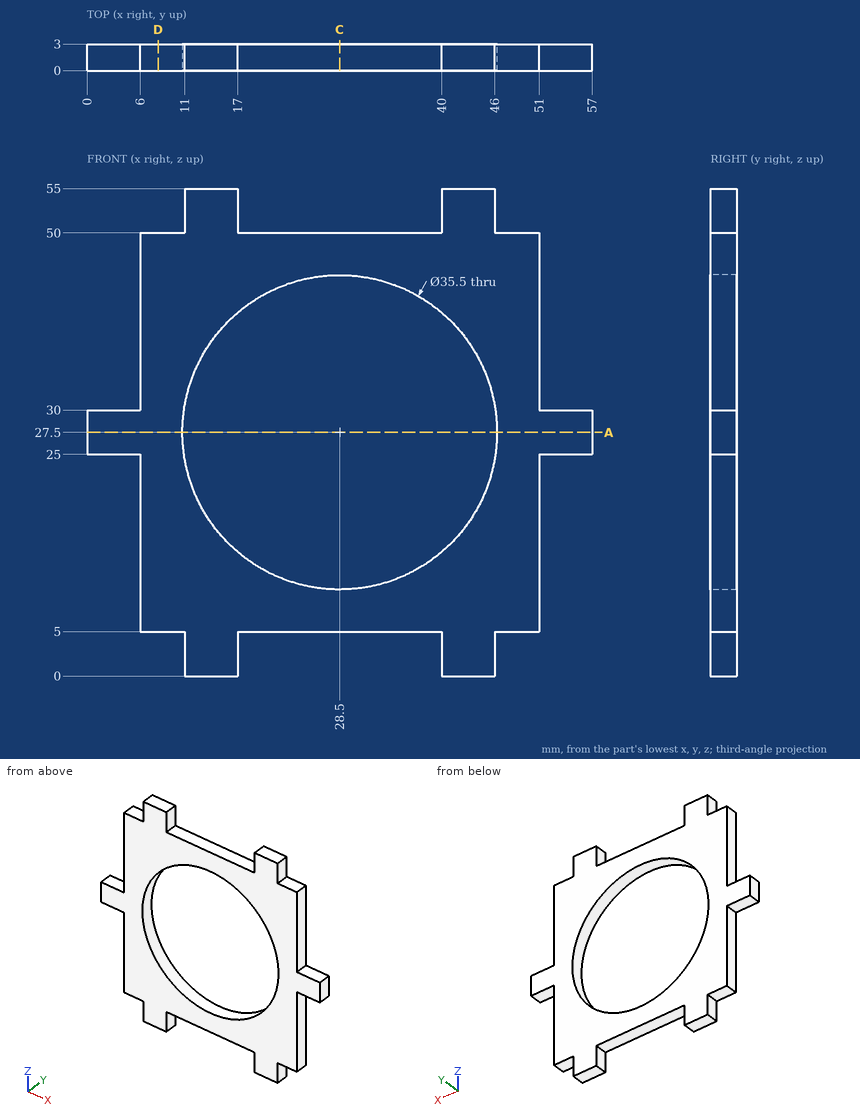
Study the drawing (mm; zero at the part's minimum x, y, z) and answer. Round coordinates to 2 decimals unless told otherwise and drop trailing zeros. Loops run counter-clockwise (first coordinate to the right, second up) from the corner with the lowest first, then second, coordinate; pieces in that order, holes last.
Q1. Given pin 1 Ø1 at (y, z) = (1, 9.5) entering from +X; pin 2 Ø0.9 at (y, z) = (2, 53.5) entering from +X; pin 3 Ø1.5 at (x, y) = (49.5, 2) entering from +Z; pin 4 Ø2 at (x, z) = (14.5, 22) entering from +Y, each flat-ended and moving along its own axis, determine where each tip first touches the part or whether it passes through.
Q2. Section D-D, the plane x = 8 is taken. Determine the outline of the cut face in (y, z).
Q3. Section C-C, the plane x = 28.5 is taken. Determine the outline of the cut face in (y, z).
Q4. Find the intervals of material crossed by line 1 (X direction, y = 0.85, z = 27.5); line 2 (Z direction, x = 28.5, y = 1.45); line 3 (Z direction, x = 4, y = 2.4), in increasing order.
Q5. Section A-A, the plane z = 27.5 is taken. Determine the outline of the cut face in (x, y).
Completed:
1. pin 1: stops at x = 51
1. pin 2: stops at x = 46
1. pin 3: stops at z = 50
1. pin 4: passes through
2. outline: (0, 5) - (3, 5) - (3, 50) - (0, 50) - close
3. outline: (0, 5) - (3, 5) - (3, 9.75) - (0, 9.75) - close; (0, 45.25) - (3, 45.25) - (3, 50) - (0, 50) - close
4. line 1: x = 0 to 10.75, 46.25 to 57
4. line 2: z = 5 to 9.75, 45.25 to 50
4. line 3: z = 25 to 30
5. outline: (0, 0) - (10.75, 0) - (10.75, 3) - (0, 3) - close; (46.25, 0) - (57, 0) - (57, 3) - (46.25, 3) - close
